```python
from build123d import *

# Parameters (mm, degrees)
F0_W      = 40
F0_H      = 20
F1_DEPTH  = 10
F2_R      = 2.1
F2_R_2    = 1.25
F3_DEPTH  = 5
F4_R      = 1
F6_DEPTH  = 25
F8_DEPTH  = 7
F10_DEPTH = 1.75
F9_R      = 2.1
F9_R_2    = 1.25
F11_DEPTH = 23
F12_R     = 1.25
F13_DEPTH = 5
F14_SIZE  = 0.25
F15_DEPTH = 30
F16_DEPTH = 16


# Not quite as in the source:
# - a feature names something its author has since deleted; it is built from what else it names


with BuildPart() as f1:
    # F0 (on Top) → F1 (new body)
    with BuildSketch(Plane.XY):
        with Locations((20, -10)):
            Rectangle(F0_W, F0_H)
    extrude(amount=F1_DEPTH)

    # F2 (on face) → F3 (cut)
    with BuildSketch(Plane.XZ.offset(20)):
        with Locations((28.5, 5)):
            Circle(F2_R)
        with Locations((28.5, 5)):
            Circle(F2_R_2, mode=Mode.SUBTRACT)
        with Locations((17.5, 5)):
            Circle(F2_R)
        with Locations((17.5, 5)):
            Circle(F2_R_2, mode=Mode.SUBTRACT)
    extrude(amount=-F3_DEPTH, mode=Mode.SUBTRACT)

    # F4 (on face) → F6 (cut)
    with BuildSketch(Plane.XY.offset(10)):
        with Locations((13, -17)):
            Circle(F4_R)
        with Locations((37, -3)):
            Circle(F4_R)
    extrude(amount=-F6_DEPTH, mode=Mode.SUBTRACT)

    # F7 (on face) → F8 (cut)
    with BuildSketch(Plane(origin=(0, 0, 0), x_dir=(1, 0, 0), z_dir=(0, 0, -1))):
        with BuildLine():
            Line((16.25, 11.25), (15.5, 11.25))
            ThreePointArc((15.5, 11.25), (14.25, 10), (15.5, 8.75))
            Line((15.5, 8.75), (16.25, 8.75))
            ThreePointArc((16.25, 8.75), (17.5, 10), (16.25, 11.25))
        make_face()
        with BuildLine():
            Line((27.25, 11.25), (26.5, 11.25))
            ThreePointArc((26.5, 11.25), (25.25, 10), (26.5, 8.75))
            Line((26.5, 8.75), (27.25, 8.75))
            ThreePointArc((27.25, 8.75), (28.5, 10), (27.25, 11.25))
        make_face()
    extrude(amount=-F8_DEPTH, mode=Mode.SUBTRACT)

    # F4 (on face) → F10 (cut)
    with BuildSketch(Plane.XY.offset(10)):
        with BuildLine():
            Line((15.125, -20), (15.125, -16))
            ThreePointArc((15.125, -16), (13, -13.875), (10.875, -16))
            Line((10.875, -16), (10.875, -20))
            Line((10.875, -20), (15.125, -20))
        make_face()
        with Locations((13, -17)):
            Circle(F4_R, mode=Mode.SUBTRACT)
        with BuildLine():
            Line((37, -6.125), (40, -6.125))
            Line((40, -6.125), (40, 0))
            Line((40, 0), (34.875, 0))
            Line((34.875, 0), (34.875, -4))
            ThreePointArc((34.875, -4), (35.49739809, -5.50260191), (37, -6.125))
        make_face()
        with Locations((37, -3)):
            Circle(F4_R, mode=Mode.SUBTRACT)
    extrude(amount=-F10_DEPTH, mode=Mode.SUBTRACT)

    # F9 (on face) → F11 (cut)
    with BuildSketch(Plane(origin=(0, 0, 0), x_dir=(0, -1, 0), z_dir=(-1, 0, 0))):
        with Locations((5, 5)):
            Circle(F9_R)
        with Locations((5, 5)):
            Circle(F9_R_2, mode=Mode.SUBTRACT)
    extrude(amount=-F11_DEPTH, mode=Mode.SUBTRACT)

    # F12 (on face) → F13 (cut)
    with BuildSketch(Plane.XY.offset(10)):
        with Locations((7, -10)):
            Circle(F12_R)
        with Locations((33, -10)):
            Circle(F12_R)
    extrude(amount=-F13_DEPTH, mode=Mode.SUBTRACT)

    # F14
    f14_edges = [f1.edges().sort_by_distance(p)[0] for p in [
        (15.4, -20, 5),
        (26.4, -20, 5),
        (0, 0, 5),
        (0, -20, 5),
        (34.875, -2, 10),
        (17.4375, 0, 10),
        (35.497398, -5.502602, 10),
        (0, -10, 10),
        (38.5, -6.125, 10),
        (5.4375, -20, 10),
        (40, -13.0625, 10),
        (10.875, -18, 10),
        (27.5625, -20, 10),
        (13, -13.875, 10),
        (15.125, -18, 10),
        (5.75, -10, 10),
        (31.75, -10, 10),
        (0, -10, 0),
        (40, -20, 5),
        (40, 0, 4.125),
        (0, -2.9, 5),
    ]]
    chamfer(f14_edges, length=F14_SIZE)

    # F15 (cut): a face of the model
    f15_faces = [f1.faces().sort_by_distance(p)[0] for p in [
        (0, -5, 5),
    ]]
    extrude(f15_faces, amount=-F15_DEPTH, mode=Mode.SUBTRACT)

    # F16 (cut): faces of the model
    f16_faces = [f1.faces().sort_by_distance(p)[0] for p in [
        (17.5, -20, 5),
        (28.5, -20, 5),
    ]]
    extrude(f16_faces, amount=-F16_DEPTH, mode=Mode.SUBTRACT)


solid = f1.part
```
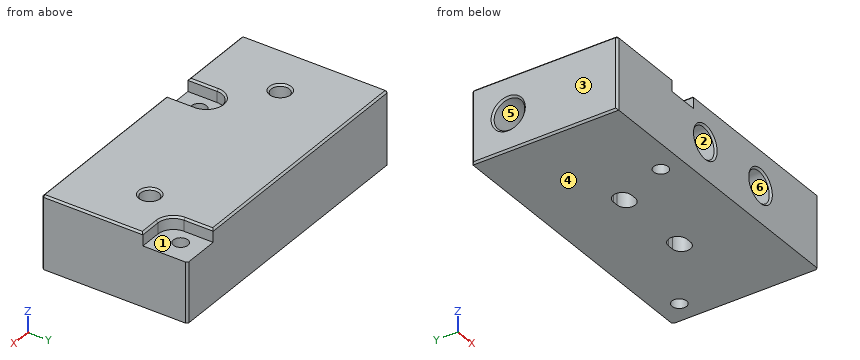
Can you work these out from the model? Positions are in its coordinate system, mm. Face numbers are marked on the shaded views. A direction names the side the tool comes from. Give positions to 0.01 mm unless a question says otherwise; leave off trailing zeros. Loops run counter-clockwise (first coordinate to the right, second up) from the corner with the lowest first, then second, coordinate; pieces in that order, holes last. Notation, with made-up numbers: M 6,16 L 48,16 A22 cw 48,42 Z; hole C 53.25,21 d4. An arc over 180 degrees is marked long. Use CSV: the item, a comma, the result in double quotes. Start each with the question number.
1. If I drill on L1, parallel to Z at x = 25.5, y = -5; L2, parallel to Z at x = 17.5, y = -17.9; L3, parallel to Y at x = 33, z = 8.25, over which ranges is the centre line in solid material (lowest first)?
2. On a 3-axis mill with a long thin cutter (end or side, diameter ignored), from which of +Z, -Z, +X, -X, +Y, -Y can I reach the whole of each face in a straight line? I mean the marked faces 4, 5 and 6. Say none if no direction works.
3. If we mould it in two halves opening along Z, with no side actions, what happens to the marked faces 1, 2 and 3? For each: released by +Z, released by -Z, zero draft, split by the parting line, or undercut.
4. Imagine slicing it at B-B, the plane x = 9. Write out the boundary of the cut face in (y, z), plus the area to 3 significant figures.
5. For P1, Ø1.6, axis at x = 13, y = -17, coming from the -Z side; P2, Ø1.3, axis at x = 18, z = 5, coming from the -Y side; P3, Ø4, axis at x = 17.5, z = 5, coming from the -Y side, each with a flat end and sliding along its axis, tell me the tip position at first contact or that it passes through.
6. Imagine slicing it at C-C, the plane x = 33. Write out the boundary of the cut face in (y, z).
7. Imagine slicing it at A-A, the plane z = 1.25. Write out the boundary of the cut face in (x, y), plus the area to 3 significant figures.
Response values:
1,L1,"0 to 3.75, 6.25 to 10"
1,L2,"0 to 2.9, 7.1 to 10"
1,L3,"-20 to -11.25, -8.75 to 0"
2,face 4,"-Z, +X, -X, +Y, -Y"
2,face 5,"-X"
2,face 6,"-Y"
3,face 1,"released by +Z"
3,face 2,"undercut"
3,face 3,"zero draft"
4,outline,"M -20,0 L 0,0 L 0,9.75 L -0.25,10 L -19.75,10 L -20,9.75 Z; hole C -5,5 d4.2"
4,area,"186 mm^2"
5,P1,"through"
5,P2,"y = -3"
5,P3,"y = -15"
6,outline,"M -20,0 L 0,0 L 0,9.75 L -0.25,10 L -8.5,10 L -8.75,9.75 L -8.75,5 L -11.25,5 L -11.25,9.75 L -11.5,10 L -19.75,10 L -20,9.75 Z"
7,outline,"M 0,-19.75 L 0.25,-20 L 39.75,-20 L 40,-19.75 L 40,-0.25 L 39.75,0 L 0.25,0 L 0,-0.25 Z; hole C 13,-17 d2; hole M 15.5,-11.25 L 16.25,-11.25 A1.25 ccw 16.25,-8.75 L 15.5,-8.75 A1.25 ccw Z; hole M 26.5,-11.25 L 27.25,-11.25 A1.25 ccw 27.25,-8.75 L 26.5,-8.75 A1.25 ccw Z; hole C 37,-3 d2"
7,area,"780 mm^2"
